For this review, take the finished solid that the model builds, in its own axes (mm). A direction names the side the tool comes from. Round coordinates to 2 decimals unless told otherwise and drop trailing zeros. Loops run counter-clockwise (first coordinate to the right, second up) from the corner with the lowest first, then second, coordinate; pieces in that order, holes last.
```python
from build123d import *

# Parameters (mm, degrees)
SKETCH1_W                                    = 32
SKETCH1_H                                    = 18
SKETCH1_R                                    = 2
BOSS_EXTRUDE1_DEPTH                          = 3
SKETCH3_W                                    = 4
SKETCH3_H                                    = 18
BOSS_EXTRUDE2_DEPTH                          = 6
SKETCH4_R                                    = 1.25
CUT_EXTRUDE1_DEPTH                           = 25.103941586
CSK_FOR_M4_HEX_SOCKET_COUNTERSUNK_HE_2_COUNT = 2
CSK_FOR_M4_HEX_SOCKET_COUNTERSUNK_HE_2_PITCH = 20


with BuildPart() as part:
    # Sketch1 → Boss-Extrude1 (new body)
    with BuildSketch(Plane(origin=(0, 0, 0), x_dir=(0, 0, -1), z_dir=(1, 0, 0))):
        Rectangle(SKETCH1_W, SKETCH1_H)
        with Locations((-10, 0)):
            Circle(SKETCH1_R, mode=Mode.SUBTRACT)
        Circle(SKETCH1_R, mode=Mode.SUBTRACT)
        with Locations((10, 0)):
            Circle(SKETCH1_R, mode=Mode.SUBTRACT)
    extrude(amount=BOSS_EXTRUDE1_DEPTH)

    # Sketch3 → Boss-Extrude2 (add)
    with BuildSketch(Plane.XY.offset(16)):
        with Locations((1, 0)):
            Rectangle(SKETCH3_W, SKETCH3_H)
    extrude(amount=BOSS_EXTRUDE2_DEPTH)

    # Sketch4 → Cut-Extrude1 (cut, through all)
    with BuildSketch(Plane(origin=(3, 0, 0), x_dir=(0, 0, -1), z_dir=(1, 0, 0))):
        with Locations((-19, -6)):
            Circle(SKETCH4_R)
    extrude(amount=-CUT_EXTRUDE1_DEPTH, mode=Mode.SUBTRACT)

    # Sketch5 → CSK for M4 Hex Socket Countersunk Head Screw1 (revolve, cut)
    with BuildSketch(Plane(origin=(3, 0, 10), x_dir=(0, 0, -1), z_dir=(0, 1, 0))):
        Polygon((0, 0), (0, 4.000025), (2.25, 4.000025), (2.25, 2.84), (5.09, 0), align=None)
    csk_for_m4_hex_socket_countersunk_head_s = revolve(axis=Axis((9.35, 0, 10), (-1, 0, 0)), mode=Mode.SUBTRACT)

    # CSK for M4 Hex Socket Countersunk He 2: CSK for M4 Hex Socket Countersunk Head Screw1 ×2
    with Locations(*[(0, 0, -i * CSK_FOR_M4_HEX_SOCKET_COUNTERSUNK_HE_2_PITCH) for i in range(1, CSK_FOR_M4_HEX_SOCKET_COUNTERSUNK_HE_2_COUNT)]):
        add(csk_for_m4_hex_socket_countersunk_head_s, mode=Mode.SUBTRACT)


solid = part.part
```
(1) For faces 4 (the flat face through (0, 0, 4)), 5 (the cylindrical face through (1.028, -6.479, 17.845)), list the 3-axis set-ups (+Z, -Z, +X, -X, +Y, -Y) from which the entire face can be reached by the end or side of a thin tool; tool diameter is ignored.
(2) For L1, parallel to Z at x = 2.1, y = -2.5; L2, parallel to Y at x = 0.1, z = -10; L3, parallel to Z at x = 2.15, y = -0.5, list the stretches that pass through material, from the lowest coordinate up.
(3) The part is to be moulded in two halves that separate along Z. For faces 1 (the flat face through (3, 0, 3)), 2 (the cylindrical face through (1, -2, 0)), 3 (the flat face through (-0.5, 0.1, 16)), say which applies: pulls with the +Z half, pulls with the -Z half, needs draft (parallel to the pull), parting line crosses it, or undercut.
(4) Add section C-C (y = -6). Give the boundary of the cut face in (x, z), plus the area to 3 significant figures.
(5) Insertion check: pin 1 Ø0.5 at (x, y) = (-0.5, -3.5) entering from -Z; pin 2 Ø6 at (y, z) = (0, -10) entering from -X. Each pin has a flat end and moves straight along its axis. Give the tip position at first contact, or say it passes through.
(6) Add section D-D (y = 7). Give the boundary of the cut face in (x, z), plus the area to 3 significant figures.
(7) Add section B-B (x = 1.65). Give the boundary of the cut face in (y, z), plus the area to 3 significant figures.
(8) Add section A-A (z = -10). Give the boundary of the cut face in (x, y), plus the area to 3 significant figures.
Outcome:
1. face 4: -Z, -X, +Y, -Y
1. face 5: +X, -X
2. L1: z = -16 to -13.36, -6.64 to 6.64, 13.36 to 22
2. L2: y = -9 to -2.25, 2.25 to 9
2. L3: z = -16 to -14.21, -5.79 to -1.94, 1.94 to 5.79, 14.21 to 22
3. face 1: needs draft
3. face 2: undercut
3. face 3: pulls with the -Z half
4. outline: (-1, 16) - (0, 16) - (0, -16) - (3, -16) - (3, 17.75) - (-1, 17.75) - close; (-1, 20.25) - (3, 20.25) - (3, 22) - (-1, 22) - close
4. area: 110 mm2
5. pin 1: stops at z = 16
5. pin 2: stops at x = 0
6. outline: (-1, 16) - (0, 16) - (0, -16) - (3, -16) - (3, 22) - (-1, 22) - close
6. area: 120 mm2
7. outline: (-9, -16) - (9, -16) - (9, 22) - (-9, 22) - close; hole circle Ø2.5 at (-6, 19); hole circle Ø7.48 at (0, -10); hole circle Ø7.48 at (0, 10); hole circle Ø4 at (0, 0)
7. area: 579 mm2
8. outline: (0, -9) - (3, -9) - (3, -5.09) - (0.16, -2.25) - (0, -2.25) - close; (0, 2.25) - (0.16, 2.25) - (3, 5.09) - (3, 9) - (0, 9) - close
8. area: 32.4 mm2
